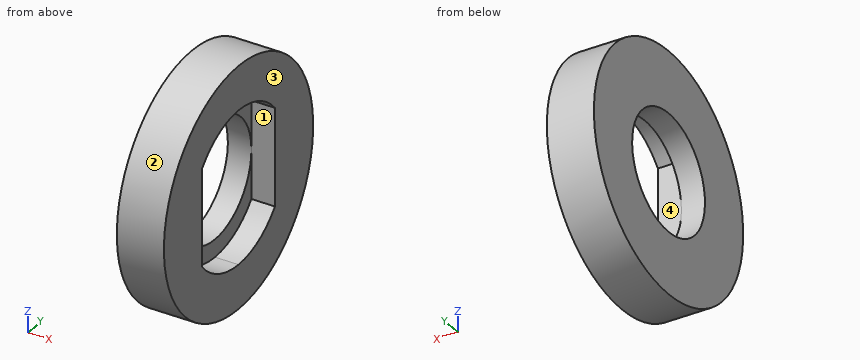
from build123d import *

# Parameters (mm, degrees)
SKETCH1_R           = 10.25
BOSS_EXTRUDE1_DEPTH = 4
SKETCH2_W           = 8.306623862
SKETCH2_H           = 10
CUT_EXTRUDE1_DEPTH  = 2
SKETCH3_R           = 5
CUT_EXTRUDE2_DEPTH  = 3


with BuildPart() as part:
    # Sketch1 → Boss-Extrude1 (new body)
    with BuildSketch(Plane(origin=(0, 0, 0), x_dir=(0, 0, -1), z_dir=(1, 0, 0))):
        Circle(SKETCH1_R)
    extrude(amount=BOSS_EXTRUDE1_DEPTH)

    # Sketch2 → Cut-Extrude1 (cut)
    with BuildSketch(Plane(origin=(4, 0, 0), x_dir=(0, 0, -1), z_dir=(1, 0, 0))):
        with BuildLine():
            ThreePointArc((-4.153311931, 5), (-6.5, 0), (-4.153311931, -5))
            Line((-4.153311931, -5), (-4.153311931, 5))
        make_face()
        Rectangle(SKETCH2_W, SKETCH2_H)
        with BuildLine():
            Line((4.153311931, 5), (4.153311931, -5))
            ThreePointArc((4.153311931, -5), (5.884153616, -2.761654617), (6.5, 0))
            ThreePointArc((6.5, 0), (5.884153616, 2.761654617), (4.153311931, 5))
        make_face()
    extrude(amount=-CUT_EXTRUDE1_DEPTH, mode=Mode.SUBTRACT)

    # Sketch3 → Cut-Extrude2 (cut, through all)
    with BuildSketch(Plane(origin=(2, 0, 0), x_dir=(0, 0, -1), z_dir=(1, 0, 0))):
        Circle(SKETCH3_R)
    extrude(amount=-CUT_EXTRUDE2_DEPTH, mode=Mode.SUBTRACT)


solid = part.part
Geometry check sheet. Reference: the model listing, model coordinates, mm. Face numbers are marked on the shaded views. Coordinates: 2 decimals unless noted, no trailing zeros. Order: outer loops, then holes, each group sorted by start corner. A loop starts at its lowest first (then second) coordinate and runs counter-clockwise, first axis right, second up. Notation, with made-up numbers: (-36.75, 85.5) - (-15.75, 85.5) arc R17 ccw to (-15.75, 109.5) - close; hole circle Ø3 at (11, -8). An arc over 180 degrees is marked (long way). Answer in a Markdown table with one row per item. Add a question column.
1) Cross-section at C-C, the plane z = -2.25. Record the cut outline in (x, y).
2) Cross-section at A-A, the plane x = 2.85. Record the cut outline in (y, z).
3) Material ranges on line 1 along Y through (x, z) = (1.3, 0); line 2 along Z through (x, y) = (2.6, 0.25); line 3 along Z through (x, y) = (2.05, -3), recorded low to high. Write a range as [from, to].
4) Gauge pin test, flat ends, axial feed: P1, Ø4, axis at y = 2.5, z = -0.5, coming from the -X side; P2, Ø2, axis at x = 1.5, z = -6, coming from the +Y side; P3, Ø8, axis at y = 6, z = -8, coming from the -X side. Record the tip position at first contact, or that the pin passes through.
5) Cross-section at D-D, the plane x = 1.3. Record the cut outline in (y, z), then the cut area to 3 significant figures.
6) Cross-section at B-B, the plane y = -3.25. Record the cut outline in (x, z), then the cut area to 3 significant figures.
7) Release check for a two-part mould opening along Z. For the marked faces 1, 2, 3 and 4 record: +Z half, -Z half, draft (parallel to the pull), parting line (faces both ways), or undercut.
Check result:
| question | item | result |
|---|---|---|
| 1 | outline | (0, -10) - (4, -10) - (4, -5) - (2, -5) - (2, -4.47) - (0, -4.47) - close; (0, 4.47) - (2, 4.47) - (2, 5) - (4, 5) - (4, 10) - (0, 10) - close |
| 2 | outline | circle Ø20.5 at (0, 0); hole (-5, -4.15) arc R6.5 ccw to (5, -4.15) - (5, 4.15) arc R6.5 ccw to (-5, 4.15) - close |
| 3 | line 1 | y = [-10.25, -5], [5, 10.25] |
| 3 | line 2 | z = [-10.25, -6.5], [6.5, 10.25] |
| 3 | line 3 | z = [-9.8, -5.77], [5.77, 9.8] |
| 4 | P1 | passes through |
| 4 | P2 | stops at y = 8.95 |
| 4 | P3 | stops at x = 0 |
| 5 | outline | circle Ø20.5 at (0, 0); hole circle Ø10 at (0, 0) |
| 5 | area | 252 mm² |
| 6 | outline | (0, -9.72) - (4, -9.72) - (4, -5.63) - (2, -5.63) - (2, -3.8) - (0, -3.8) - close; (0, 3.8) - (2, 3.8) - (2, 5.63) - (4, 5.63) - (4, 9.72) - (0, 9.72) - close |
| 6 | area | 40.1 mm² |
| 7 | face 1 | undercut |
| 7 | face 2 | parting line |
| 7 | face 3 | draft |
| 7 | face 4 | undercut |
